For this review, take the finished solid that the model builds, in its own axes (mm). Face numbers are marked on the shaded views. A direction names the side the tool comes from. Coordinates: 2 decimals unless noted, no trailing zeros. Order: outer loops, then holes, each group sorted by start corner. A loop starts at its lowest first (then second) coordinate and runs counter-clockwise, first axis right, second up. Notation, with made-up numbers: M -22,74.25 L -1,74.25 A32 cw -1,101.25 Z; hole C 59.25,32 d11. An arc over 180 degrees is marked long. Use CSV: the item, a comma, the result in double quotes.
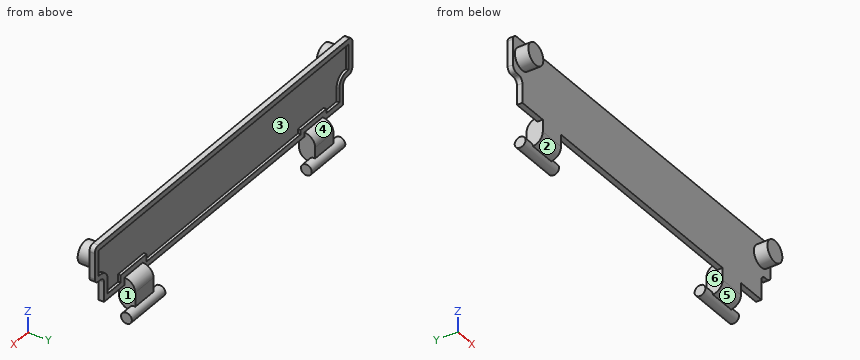
```python
from build123d import *

# Parameters (mm, degrees)
SKETCH1_R                = 2
BOSS_EXTRUDE1_DEPTH      = 2.5
BOSS_EXTRUDE1_2_DEPTH    = 2.5
BOSS_EXTRUDE3_DEPTH      = 1
FILLET1_R                = 1
BOSS_EXTRUDE4_DEPTH      = 2
BOSS_EXTRUDE4_DEPTH_BACK = 1
SKETCH3_W                = 4.9
SKETCH3_H                = 5.030022666
SKETCH3_H_2              = 5.609354891
BOSS_EXTRUDE5_DEPTH      = 2
BOSS_EXTRUDE5_DEPTH_BACK = 7
SKETCH4_R                = 1
BOSS_EXTRUDE6_DEPTH      = 2
BOSS_EXTRUDE6_DEPTH_BACK = 7
SKETCH5_R                = 1
FILLET2_R                = 2
FILLET3_R                = 2
CUT_EXTRUDE1_DEPTH       = 0.5
FILLET4_R                = 2


# Some blends are built 0.0001 mm under size
with BuildPart() as part:
    # Sketch1 → Boss-Extrude1 (new body)
    with BuildSketch(Plane(origin=(0, 0, 0), x_dir=(1, 0, 0), z_dir=(0, 1, 0))):
        with Locations(Location((64.1, 0, 0), (0, 0, 270))):
            Circle(SKETCH1_R)
    extrude(amount=BOSS_EXTRUDE1_DEPTH)



with BuildPart() as body_2:
    # Sketch1 → Boss-Extrude1 2 (new body)
    with BuildSketch(Plane(origin=(0, 0, 0), x_dir=(1, 0, 0), z_dir=(0, 1, 0))):
        with Locations(Location((0, 0, 0), (0, 0, 270))):
            Circle(SKETCH1_R)
    extrude(amount=BOSS_EXTRUDE1_2_DEPTH)


with BuildPart() as part_1:
    add(part.part)

    add(body_2.part)  # Boss-Extrude3 merges body 2
    # Sketch2 → Boss-Extrude3 (add)
    with BuildSketch(Plane(origin=(0, 2.5, 0), x_dir=(1, 0, 0), z_dir=(0, 1, 0))):
        Polygon((0, 3.373067478), (0, 8), (64.1, 8), (64.1, 3.373067478), (66.585371827, 3.373067478), (66.585371827, -3.373067478), (-2.485371827, -3.373067478), (-2.485371827, 3.373067478), align=None)
    extrude(amount=BOSS_EXTRUDE3_DEPTH)

    # Fillet1
    fillet1_edges = [part_1.edges().sort_by_distance(p)[0] for p in [
        (64.1, 3, -3.373067478),
        (0, 3, -3.373067478),
        (-2.485371827, 3, -3.373067478),
        (-2.485371827, 3, 3.373067478),
        (66.585371827, 3, 3.373067478),
        (66.585371827, 3, -3.373067478),
    ]]
    fillet(fillet1_edges, radius=FILLET1_R)

    # Sketch3 → Boss-Extrude4 (add, two sides: drawn at the far end of the back side and taken through both)
    with BuildSketch(Plane(origin=(0, 3.5, 0), x_dir=(1, 0, 0), z_dir=(0, 1, 0)).offset(-BOSS_EXTRUDE4_DEPTH_BACK)):
        with Locations((7.93, 9.710321272)):
            Rectangle(SKETCH3_W, SKETCH3_H)
        with Locations((56.17, 9.42065516)):
            Rectangle(SKETCH3_W, SKETCH3_H_2)
    extrude(amount=BOSS_EXTRUDE4_DEPTH + BOSS_EXTRUDE4_DEPTH_BACK)

    # Sketch4 → Boss-Extrude5 (add, two sides: drawn at the far end of the back side and taken through both)
    with BuildSketch(Plane.ZY.offset(-5.48).offset(-BOSS_EXTRUDE5_DEPTH_BACK)):
        with Locations((-12.225332605, 5.316497078)):
            Circle(SKETCH4_R)
    extrude(amount=BOSS_EXTRUDE5_DEPTH + BOSS_EXTRUDE5_DEPTH_BACK)

    # Sketch5 → Boss-Extrude6 (add, two sides: drawn at the far end of the back side and taken through both)
    with BuildSketch(Plane.ZY.offset(-53.72).offset(-BOSS_EXTRUDE6_DEPTH_BACK)):
        with Locations((-12.225332605, 5.316497078)):
            Circle(SKETCH5_R)
    extrude(amount=BOSS_EXTRUDE6_DEPTH + BOSS_EXTRUDE6_DEPTH_BACK)

    # Fillet2
    fillet2_edges = [part_1.edges().sort_by_distance(p)[0] for p in [
        (56.17, 5.5, -6.615977714),
        (7.93, 5.5, -7.195309939),
    ]]
    fillet(fillet2_edges, radius=FILLET2_R - 0.0001)  # a hair under: the kernel refuses the full size

    # Fillet3
    # the kernel refuses this fillet: 2 mm, written as the material it takes off along each edge
    with BuildSketch(Plane(origin=(48.741090307, 2.5, -12.225332605), x_dir=(0, 0, 1), z_dir=(1, 0, 0))) as fillet3_piece_1:
        with BuildLine():
            CenterArc((1.991563877, -2), FILLET3_R, 90, 84.735624625)
            Line((0, -1.816497078), (-0.039831278, -1.81282702))
            ThreePointArc((-0.039831278, -1.81282702), (-0.04, -0.908248539), (-0.04, 0))
            Line((-0.04, 0), (0, 0.04))
            Line((0, 0.04), (1.991563877, 0.04))
            Line((1.991563877, 0.04), (1.991563877, 0))
        make_face()
    extrude(amount=14.857819387, mode=Mode.SUBTRACT)

    # Sketch6 → Cut-Extrude1 (cut)
    with BuildSketch(Plane(origin=(0, 3.5, 0), x_dir=(1, 0, 0), z_dir=(0, 1, 0))):
        with BuildLine():
            Line((59.62, 5.615977714), (52.72, 5.615977714))
            Line((52.72, 5.615977714), (52.72, 7))
            Line((52.72, 7), (11.38, 7))
            Line((11.38, 7), (11.38, 6.195309939))
            Line((11.38, 6.195309939), (4.48, 6.195309939))
            Line((4.48, 6.195309939), (4.48, 7))
            Line((4.48, 7), (1, 7))
            Line((1, 7), (1, 4.373067478))
            ThreePointArc((1, 4.373067478), (0.414213562, 2.958853916), (-1, 2.373067478))
            Line((-1, 2.373067478), (-1.485371827, 2.373067478))
            Line((-1.485371827, 2.373067478), (-1.485371827, -2.373067478))
            Line((-1.485371827, -2.373067478), (65.585371827, -2.373067478))
            Line((65.585371827, -2.373067478), (65.585371827, 2.373067478))
            Line((65.585371827, 2.373067478), (65.1, 2.373067478))
            ThreePointArc((65.1, 2.373067478), (63.685786438, 2.958853916), (63.1, 4.373067478))
            Line((63.1, 4.373067478), (63.1, 7))
            Line((63.1, 7), (59.62, 7))
            Line((59.62, 7), (59.62, 5.615977714))
        make_face()
    extrude(amount=-CUT_EXTRUDE1_DEPTH, mode=Mode.SUBTRACT)

    # Fillet4
    # the kernel refuses this fillet: 2 mm, written as the material it takes off along each edge
    with BuildSketch(Plane(origin=(15.358909693, 2.5, -12.225332605), x_dir=(0, 0, 1), z_dir=(-1, 0, 0))) as fillet4_piece_1:
        with BuildLine():
            CenterArc((1.991563877, 2), FILLET4_R, 185.264375375, 84.735624625)
            Line((0, 1.816497078), (-0.039831278, 1.81282702))
            ThreePointArc((-0.039831278, 1.81282702), (-0.04, 0.908248539), (-0.04, 0))
            Line((-0.04, 0), (0, -0.04))
            Line((0, -0.04), (1.991563877, -0.04))
            Line((1.991563877, -0.04), (1.991563877, 0))
        make_face()
    extrude(amount=14.857819387, mode=Mode.SUBTRACT)


solid = part_1.part
```
Item 1: Add section A-A on x = 26.5. State the section outline as (y, z) points.
Solutions:
outline,"M 2.5,-8 L 3.5,-8 L 3.5,-7 L 3,-7 L 3,2.37 L 3.5,2.37 L 3.5,3.37 L 2.5,3.37 Z"
Item 2: Draft analysis for pull direction Z (two halves, no side actions). For the marked faces 1, 2, 3 and 4, state which applies: released by +Z, released by -Z, zero draft, split by the parting line, or undercut.
Solutions:
face 1,"zero draft"
face 2,"released by -Z"
face 3,"undercut"
face 4,"released by +Z"
Item 3: Clearance check with flat-ended pins moving along their axes: pin 1 Ø1.5 at (y, z) = (3, -8) entering from +X; pin 2 Ø2 at (x, y) = (20, 1) entering from +Z; pin 3 Ø0.6 at (y, z) = (5.5, -12) entering from -X; pin 4 Ø0.5 at (x, y) = (3.5, 3) entering from -Z. State where each tip first meets the part, or that it passes through.
Solutions:
pin 1,"x = 64.1"
pin 2,"through"
pin 3,"x = 3.48"
pin 4,"z = -8"
Item 4: To check wall thickness, follow line 1 along X through (y, z) = (4.75, -8.25); line 2 along X through (y, z) = (1.75, 0); line 3 along Y through (x, z) = (7, -10). State the ranges of each line that lie inside material, in increasing order. Write a range as [from, to].
Solutions:
line 1,"[5.48, 10.38], [53.72, 58.62]"
line 2,"[-2, 2], [62.1, 66.1]"
line 3,"[2.5, 5.5]"
Item 5: Add section B-B on z = -0.75. State the section outline as (x, y) points.
Solutions:
outline,"M -2.49,2.5 L -1.85,2.5 L -1.85,0 L 1.85,0 L 1.85,2.5 L 62.25,2.5 L 62.25,0 L 65.95,0 L 65.95,2.5 L 66.59,2.5 L 66.59,3.5 L 65.59,3.5 L 65.59,3 L -1.49,3 L -1.49,3.5 L -2.49,3.5 Z"
Item 6: For the marked faces 5 and 6, list the 3-axis set-ups (+Z, -Z, +X, -X, +Y, -Y) from which the entire face can be reached by the end or side of a thin tool; tool diameter is ignored.
Solutions:
face 5,"-Z, +X, -X, -Y"
face 6,"none"
